Geometry check sheet. Reference: the model listing, model coordinates, mm. A direction names the side the tool comes from. Round coordinates to 2 decimals unless told otherwise and drop trailing zeros. Loops run counter-clockwise (first coordinate to the right, second up) from the corner with the lowest first, then second, coordinate; pieces in that order, holes last. Notation, with made-up numbers: (-17.75, -37) - (40.25, -37) arc R26 ccw to (40.25, -11) - close; hole circle Ø10 at (58, -9.75). An arc over 180 degrees is marked (long way). Answer in a Markdown table with one row per item. Add a question column.
```python
from build123d import *

# Parameters (mm, degrees)
BOSS_EXTRUDE1_DEPTH     = 12.7
BOSS_EXTRUDE2_DEPTH     = 6.35
FILLET1_R               = 1.27
FILLET2_R               = 1.27
CUT_EXTRUDE1_DEPTH      = 52.669649941
CUT_EXTRUDE1_DEPTH_BACK = 52.669649941
SKETCH5_R               = 3.683


with BuildPart() as part:
    # Sketch1 → Boss-Extrude1 (new body)
    with BuildSketch(Plane(origin=(0, 0, 0), x_dir=(1, 0, 0), z_dir=(0, 1, 0))):
        Polygon((0, 0), (0, 31.75), (-22.86, 31.75), (-22.86, 25.4), (-6.35, 25.4), (-6.35, 0), align=None)
    extrude(amount=BOSS_EXTRUDE1_DEPTH)

    # Sketch3 → Boss-Extrude2 (add)
    with BuildSketch(Plane(origin=(0, 0, -31.75), x_dir=(-1, 0, 0), z_dir=(0, 0, -1))):
        Polygon((22.86, 12.7), (33.655, 12.7), (33.655, -3.175), (36.195, -3.175), (36.195, -0.6985), (38.735, -0.6985), (38.735, -12.0015), (36.195, -12.0015), (36.195, -9.525), (33.655, -9.525), (33.655, -12.0015), (27.305, -12.0015), (27.305, 0), (22.86, 0), align=None)
    extrude(amount=-BOSS_EXTRUDE2_DEPTH)

    # Fillet1
    fillet1_edges = [part.edges().sort_by_distance(p)[0] for p in [
        (-36.195, -0.6985, -28.575),
    ]]
    fillet(fillet1_edges, radius=FILLET1_R)

    # Fillet2
    fillet2_edges = [part.edges().sort_by_distance(p)[0] for p in [
        (-36.195, -12.0015, -28.575),
        (-38.735, -12.0015, -28.575),
        (-38.735, -0.6985, -28.575),
    ]]
    fillet(fillet2_edges, radius=FILLET2_R - 0.0001)  # a hair under: the kernel refuses the full size

    # Sketch5 → Cut-Extrude1 (cut, two sides: drawn at the far end of the back side and taken through both)
    with BuildSketch(Plane(origin=(0, 0, 0), x_dir=(0, 0, -1), z_dir=(1, 0, 0)).offset(-CUT_EXTRUDE1_DEPTH_BACK)):
        with Locations((6.223, 6.35)):
            Circle(SKETCH5_R)
    extrude(amount=CUT_EXTRUDE1_DEPTH + CUT_EXTRUDE1_DEPTH_BACK, mode=Mode.SUBTRACT)


solid = part.part
```
Q1. Set-up check for faces 1 (the flat face through (-36.195, -10, -29)), 2 (the flat face through (-36.195, -3, -29)), 3 (the cylindrical face through (-38.37, -11.62, -28.53)), 4 (the cylindrical face through (-38.35, -1.06, -28.53)), 5 (the flat face through (-23, 3, -25.4)): record each of +Z, -Z, +X, -X, +Y, -Y from which the full face is reachable in a straight line by a thin tool's end or side.
Q2. Cross-section at C-C, the plane x = -10.5. Enter the section's corners in (y, z), plus the area to 3 significant figures.
Q3. Release check for a two-part mould opening along X. For faces 6 (the flat face through (-27.305, -6, -29)), 7 (the flat face through (-31, -12.002, -29)), 8 (the cylindrical face through (-36.58, -11.64, -28.53)) record: +X half, -X half, draft (parallel to the pull), parting line (faces both ways), or undercut.
Q4. Scan lines: line 1 (Z direction, x = -30, y = 1.25); line 2 (X direction, y = 5.5, z = -14.5); line 3 (Z direction, x = -3.75, y = 6.35). Record each from-to range of solid material in increasing order. Write a range as from..to.
Q5. Cross-section at B-B, the plane z = -15.5. Enter the section's corners in (x, y), plus the area to 3 significant figures.
Q6. Cross-section at A-A, the plane y = 6.35. Enter the section's corners in (x, z) (3 decimals).
Q7. Depth check by flat-ended pin: P1, Ø2.5, axis at y = -11, z = -28, coming from the -X side (3 decimals); P2, Ø4, axis at y = 5, z = -14, coming from the -X side; P3, Ø0.8, axis at x = -35.5, z = -28, coming from the +Y side (3 decimals); P4, Ø0.6, axis at y = -2.5, z = -29.5, coming from the +X side (3 decimals). Enter the tip coordinate at first touch or a pass-through.
Check sheet entries:
| question | item | result |
|---|---|---|
| 1 | face 1 | +Z, -Z, -Y |
| 1 | face 2 | +Z, -Z, +Y |
| 1 | face 3 | +Z, -Z, -X, -Y |
| 1 | face 4 | +Z, -Z, -X, +Y |
| 1 | face 5 | +Z, -X, +Y, -Y |
| 2 | outline | (0, -31.75) - (12.7, -31.75) - (12.7, -25.4) - (0, -25.4) - close |
| 2 | area | 80.6 mm² |
| 3 | face 6 | +X half |
| 3 | face 7 | draft |
| 3 | face 8 | undercut |
| 4 | line 1 | -31.75..-25.4 |
| 4 | line 2 | -6.35..0 |
| 4 | line 3 | -31.75..-9.91, -2.54..0 |
| 5 | outline | (-6.35, 0) - (0, 0) - (0, 12.7) - (-6.35, 12.7) - close |
| 5 | area | 80.6 mm² |
| 6 | outline | (-33.655, -31.75) - (0, -31.75) - (0, -9.906) - (-6.35, -9.906) - (-6.35, -25.4) - (-33.655, -25.4) - close; (-6.35, -2.54) - (0, -2.54) - (0, 0) - (-6.35, 0) - close |
| 7 | P1 | x = -38.735 |
| 7 | P2 | x = -6.35 |
| 7 | P3 | y = -3.175 |
| 7 | P4 | x = -27.305 |
